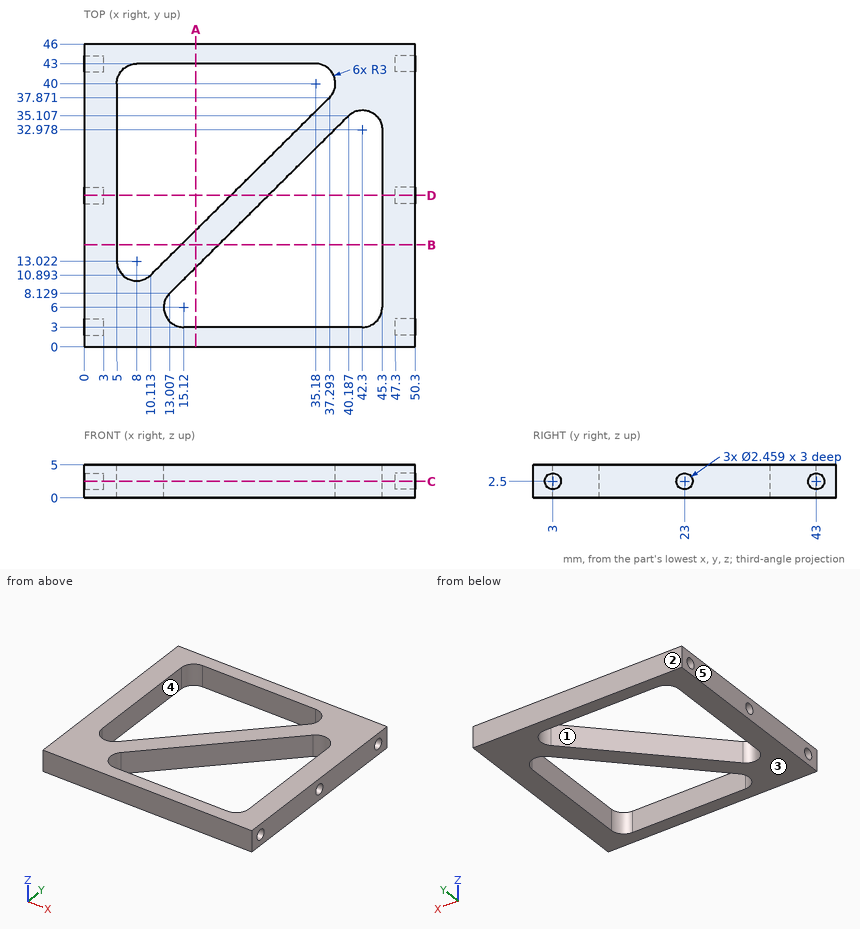
Print and shaded views of the part. All mm, measured from the part's lowest x, y and z. A direction names the side the tool comes from. Round coordinates to 2 decimals unless told otherwise and drop trailing zeros. Write each loop counter-clockwise with the first axis right and the second up, starting at its lowest first coordinate (ties: lowest second). Pieces come first, ordered by that corner, then holes.
(1) Slice it at A-A, the plane x = 17. Write the cut outline in (y, z).
(2) Slice it at B-B, the plane y = 15.5. Write the cut outline in (x, z) (1 decimal).
(3) Slice it at C-C, the plane z = 2.5. Count the separate pieces of the cut face and the enclosed holes in it, and give its area (3 significant figures).
(4) Probe line 1 along Y through (x, z) = (49.5, 2.5); line 2 along X through (y, z) = (17, 2.8) (1 decimal); line 3 along X through (y, z) = (32.5, 2.45). List the from-to ranges inside material, lowest first.
(5) Drop flat-ended pins along their axis: P1, Ø1.5, axis at y = 3, z = 2.5, coming from the -X side; P2, Ø2, axis at y = 3, z = 2.5, coming from the +X side; P3, Ø8, axis at x = 38, y = 9.5, coming from the -Z side. Give the stop position or say it passes through.
(6) Slice it at D-D, the plane y = 23. Write the cut outline in (x, z).
(7) 3-axis set-ups, long thin cutter, end or side, ignore diameter. For the marked faces 1 and 2: which of +Z, -Z, +X, -X, +Y, -Y reach the whole face in a straight line?
(8) Mould opens along X. For the marked faces 3, 4 and 5 say: pulls with the +X half, pulls with the -X half, needs draft (parallel to the pull), parting line crosses it, or undercut.
From the geometry:
1. outline: (0, 0) - (3, 0) - (3, 5) - (0, 5) - close; (12.09, 0) - (17.73, 0) - (17.73, 5) - (12.09, 5) - close; (43, 0) - (46, 0) - (46, 5) - (43, 5) - close
2. outline: (0, 0) - (5, 0) - (5, 5) - (0, 5) - close; (14.8, 0) - (20.4, 0) - (20.4, 5) - (14.8, 5) - close; (45.3, 0) - (50.3, 0) - (50.3, 5) - (45.3, 5) - close
3. separate pieces: 1
3. enclosed holes: 2
3. area: 925 mm2
4. line 1: y = 0 to 1.77, 4.23 to 21.77, 24.23 to 41.77, 44.23 to 46
4. line 2: x = 0 to 5, 16.3 to 21.9, 45.3 to 50.3
4. line 3: x = 0 to 5, 31.88 to 37.56, 45.3 to 50.3
5. P1: stops at x = 3
5. P2: stops at x = 47.3
5. P3: passes through
6. outline: (0, 0) - (5, 0) - (5, 5) - (0, 5) - (0, 3.73) - (3, 3.73) - (3, 1.27) - (0, 1.27) - close; (22.31, 0) - (27.99, 0) - (27.99, 5) - (22.31, 5) - close; (45.3, 0) - (50.3, 0) - (50.3, 1.27) - (47.3, 1.27) - (47.3, 3.73) - (50.3, 3.73) - (50.3, 5) - (45.3, 5) - close
7. face 1: +Z, -Z
7. face 2: +Z, -Z, +X, -X, +Y
8. face 3: needs draft
8. face 4: undercut
8. face 5: pulls with the -X half
